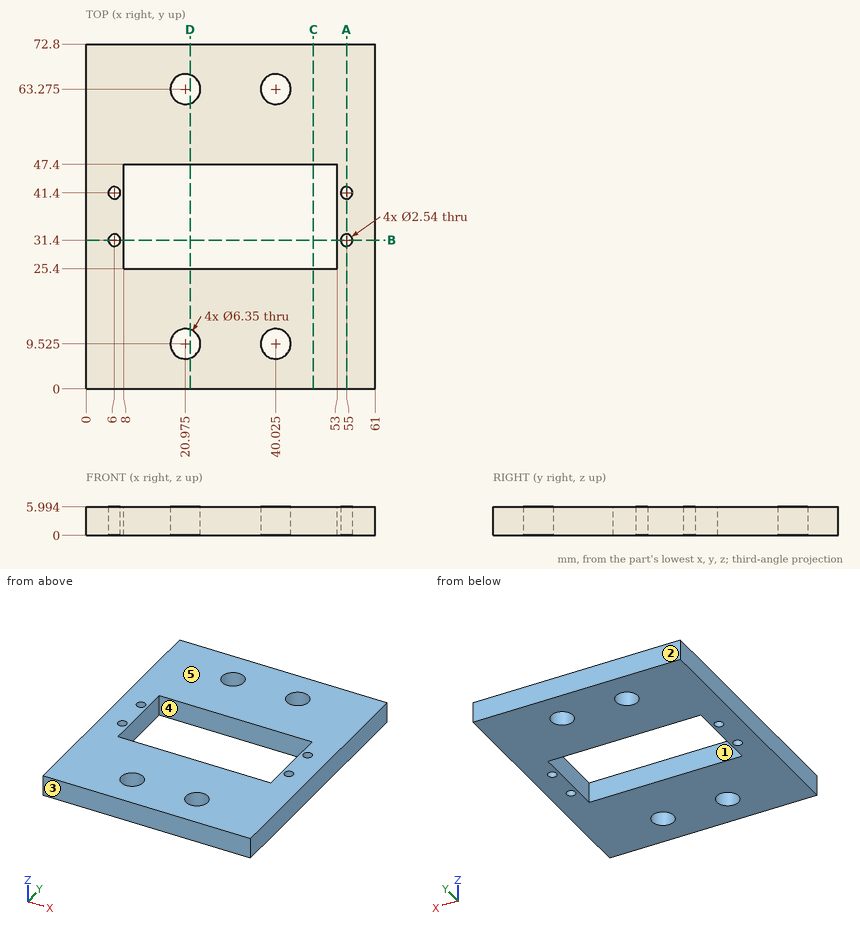
The drawing under review shows one solid part. Ordinate dimensions are in mm from its lowest x, y, z. A direction names the side the tool comes from. Coordinates: 2 decimals unless noted, no trailing zeros. Loops run counter-clockwise (first coordinate to the right, second up) from the corner with the lowest first, then second, coordinate; pieces in that order, holes last. Notation, with made-up numbers: (28.5, -25.75) - (52.5, -25.75) arc R9 ccw to (52.5, -11.75) - close; hole circle Ø3 at (3, 34.5). An arc over 180 degrees is marked (long way). Return JSON: item names as keys, results as strings.
Item 1: Take a section at D-D (x = 22). Give the boundary of the cut face in (y, z) (1 decimal).
Determined:
{"outline": "(0, 0) - (6.5, 0) - (6.5, 6) - (0, 6) - close; (12.5, 0) - (25.4, 0) - (25.4, 6) - (12.5, 6) - close; (47.4, 0) - (60.3, 0) - (60.3, 6) - (47.4, 6) - close; (66.3, 0) - (72.8, 0) - (72.8, 6) - (66.3, 6) - close"}
Item 2: Take a section at B-B (y = 31.4). Give the boundary of the cut face in (x, z) (1 decimal).
Determined:
{"outline": "(0, 0) - (4.7, 0) - (4.7, 6) - (0, 6) - close; (7.3, 0) - (8, 0) - (8, 6) - (7.3, 6) - close; (53, 0) - (53.7, 0) - (53.7, 6) - (53, 6) - close; (56.3, 0) - (61, 0) - (61, 6) - (56.3, 6) - close"}
Item 3: For the marked faces 4 and 5, list the 3-axis set-ups (+Z, -Z, +X, -X, +Y, -Y) from which the entire face can be reached by the end or side of a thin tool; tool diameter is ignored.
Determined:
{"face 4": "+Z, -Z", "face 5": "+Z, +X, -X, +Y, -Y"}
Item 4: Take a section at C-C (x = 48). Give the boundary of the cut face in (y, z) (1 decimal).
Determined:
{"outline": "(0, 0) - (25.4, 0) - (25.4, 6) - (0, 6) - close; (47.4, 0) - (72.8, 0) - (72.8, 6) - (47.4, 6) - close"}
Item 5: Take a section at A-A (x = 55). Give the boundary of the cut face in (y, z) (1 decimal), then the cut area to 3 significant figures.
Determined:
{"outline": "(0, 0) - (30.1, 0) - (30.1, 6) - (0, 6) - close; (32.7, 0) - (40.1, 0) - (40.1, 6) - (32.7, 6) - close; (42.7, 0) - (72.8, 0) - (72.8, 6) - (42.7, 6) - close", "area": "406 mm2"}
Item 6: Insertion check: pin 1 (7.5 mm diameter, centred on x = 20.975, y = 9.525, fed in from -Z). The pin has a flat end and moves straight along its axis. Give the tip position at first contact, or say it passes through.
Determined:
{"pin 1": "stops at z = 0"}
Item 7: For line 1 (Y direction, x = 55, z = 4.45); line 2 (X direction, y = 63.5, z = 1.25); line 3 (Y direction, x = 36, z = 0.9), list the stretches that pass through material, from the lowest coordinate up.
Determined:
{"line 1": "y = 0 to 30.13, 32.67 to 40.13, 42.67 to 72.8", "line 2": "x = 0 to 17.81, 24.14 to 36.86, 43.19 to 61", "line 3": "y = 0 to 25.4, 47.4 to 72.8"}
Item 8: Mouldability with a two-part tool opening along Y and no side actions: class the marked faces 1, 2 and 3 as pulls with the +Y half, pulls with the -Y half, needs draft (parallel to the pull), parting line crosses it, or undercut.
Determined:
{"face 1": "undercut", "face 2": "pulls with the +Y half", "face 3": "pulls with the -Y half"}
